Autodesk Inventor part; units mm, degrees
ref_plane "Work Plane1" through (29, 0, 0) normal (0, -1, 0) x (1, 0, 0)
ref_plane "YZ Plane" through (0, 0, 0) normal (1, 0, 0) x (0, 1, 0)
ref_plane "XZ Plane" through (0, 0, 0) normal (0, 1, 0) x (-1, 0, 0)
sketch "Sketch1" plane through (0, 0, 0) normal (0, 0, 1) x (1, 0, 0)
  line L0 (-2, 0) -> (25, 0)
  line L1 (25, 0) -> (25, 4)
  line L2 (25, 4) -> (3.125, 4)
  line L3 (3.125, 4) -> (2.3581, 4)
  line L4 (2.3581, 4) -> (0, 4)
  line L5 (0, 4) -> (0, 6.5)
  line L6 (0, 6.5) -> (-8, 6.5)
  line L7 (-8, 6.5) -> (-8, 3.4641)
  line L8 (-8, 3.4641) -> (-4, 3.4641)
  line L9 (-4, 3.4641) -> (-2, 0)
  line L10 (-14.6, 0) -> (31.6, 0)
  line L11 (0, -1.3) -> (0, 7.8)
  line L12 (3.125, 4) -> (0, 4) construction
  dimension "d1" = 21.875
  dimension "d2" = 0.7669
  dimension "d3" = 8
  dimension "d4" = 4
  dimension "d5" = 60
  dimension "d6" = 8
  dimension "d7" = 8
  dimension "d8" = 6.9282
  dimension "d9" = 13
  dimension "d26" = 25
revolve "Body" add sketch "Sketch1" angle 360 about axis through (-2, 0, 0) along (1, 0, 0)
sketch "Sketch2" plane through (-8, 0, 0) normal (-1, 0, 0) x (0, 0, 1)
  circle A0 centre (0, 0) radius 3.4641
  line L0 (0, -9.1) -> (0, 9.1)
  line L1 (-9.1, 0) -> (9.1, 0)
  line L2 (3.4641, 0) -> (1.7321, -3)
  line L3 (1.7321, -3) -> (-1.7321, -3)
  line L4 (-1.7321, -3) -> (-3.4641, 0)
  line L5 (-3.4641, 0) -> (-1.7321, 3)
  line L6 (-1.7321, 3) -> (1.7321, 3)
  line L7 (1.7321, 3) -> (3.4641, 0)
extrude "Slot" add sketch "Sketch2" against normal up to next contours L7 A0 | A0 L2 | L6 L0 A0 | A0 L0 L3 | L0 L6 A0 | A0 L3 L0 | L4 A0 | A0 L5
fillet "Fillet1" radius 0.8 1 edges at (-8, -6.5, 0)
thread "Thread"
chamfer "Chamfer1" distance 0.7668 distance2 0.7668 1 edges at (25, -4, 0) measured on face at (25, -0.6859, 0.8072)
ref_plane "Work Plane1" through (29, 0, 0) normal (0, -1, 0) x (1, 0, 0)
fillet "Fillet2" radius 0.4 1 edges at (0, -4, 0)
equation "\"d1\" = GEL"
equation "\"d3\" = KOH"
equation "\"d4\" = INTI"
equation "\"d6\" = GD"
equation "\"d7\" = BDM"
equation "\"d8\" = 1.1547 * SW"
equation "\"d9\" = KOD"
equation "\"d26\" = NLG"
equation "\"d30\" = R"
equation "\"d17\" = RR"
equation "\"d13\" = GEL"
equation "\"d15\" = -0.5 * SPD + 0.5 * GD"
equation "\"d16\" = GUL"
equation "\"GD\" = NND"
equation "\"NLG\" = 25"
equation "\"GEL\" = 21.875"
equation "\"KOD\" = 13"
equation "\"KOH\" = 8"
equation "\"INTI\" = 4"
equation "\"GAL\" = 0.61345 * PTC"
equation "\"GUL\" = 0.61345 * PTC"
equation "\"BDM\" = NND"
equation "\"SW\" = 6"
equation "\"RR\" = 0.8"
equation "\"SPD\" = NND - 1.2269 * PTC"
equation "\"R\" = 0.4"
equation "\"TOA\" = 30deg"
equation "\"GD1\" = THREADDIA - 1.2269 * PTC"
equation "\"THREADDIA\" = 8"
equation "\"FAWI\" = 45deg"
equation "\"ANG\" = 120deg"
equation "\"PTC\" = 1.25"
equation "\"NND\" = 8"
equation "\"E0\" = 1.155 * SW"
properties part number "Allen Key 8x25mm" material "Steel, Mild"
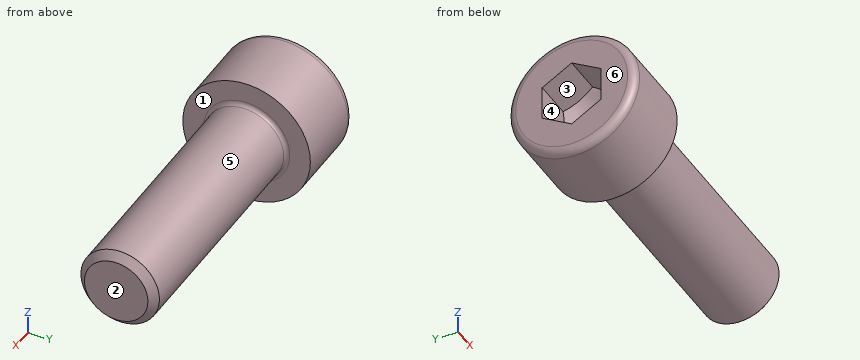
Here's how the part is built. I have some questions about the finished solid (model axes, mm). Face numbers are marked on the shaded views. A direction names the side the tool comes from. Coordinates: 2 decimals unless noted, no trailing zeros. Order: outer loops, then holes, each group sorted by start corner. A loop starts at its lowest first (then second) coordinate and runs counter-clockwise, first axis right, second up. Notation, with made-up numbers: (-7.5, 85.5) - (-0.5, 85.5) arc R24 ccw to (-0.5, 120.5) - close; hole circle Ø5 at (-16, 88). An arc over 180 degrees is marked (long way). Use CSV: the item, a comma, the result in double quotes. Start each with the question number.
1. Suppose I cut it at A-A on x = 4. List the corners of the cut face in (y, z) for me, then the cut area to 3 significant figures.
2. Please list where these lines run through material, in increasing order: line 1 (X direction, y = -1.5, z = -4.25); line 2 (Y direction, x = -3, z = -0.75); line 3 (Y direction, x = -4, z = 2). Write a range as from..to.
3. I'm going to push flat-ended pins straight in: pin 1 (1.7 mm diameter, centred on x = -6.5, z = -0.5, fed in from +Y); pin 2 (1.5 mm diameter, centred on x = 6, y = -2.5, fed in from -Z); pin 3 (1 mm diameter, centred on y = 3, z = -4, fed in from +X); pin 4 (2 mm diameter, centred on x = -4, y = 3.5, fed in from +Z). Where does each tip first touch, or does it pass through?
4. If we mould it in two halves opening along Y, with no side actions, what happens to the marked faces 4, 5 and 6? For each: +Y half, -Y half, draft (parallel to the pull), parting line (faces both ways), or undercut.
5. For the marked faces 1, 2 and 3, which set-ups out of +Z, -Z, +X, -X, +Y, -Y let a thin tool reach every point of the face, with its end or its side?
Output:
1,outline,"circle Ø8 at (0, 0)"
1,area,"50.3 mm2"
2,line 1,"x = -8..0"
2,line 2,"y = -6.46..-1.56, 1.56..6.46"
2,line 3,"y = -6.18..-2.54, 2.54..6.18"
3,pin 1,"stops at y = 6.5"
3,pin 2,"stops at z = -3.6"
3,pin 3,"stops at x = 0"
3,pin 4,"stops at z = 6"
4,face 4,"undercut"
4,face 5,"parting line"
4,face 6,"draft"
5,face 1,"+X"
5,face 2,"+Z, -Z, +X, +Y, -Y"
5,face 3,"-X"
